Could you check a few things on this model? Use its own coordinates, in mm. A direction names the side the tool comes from. Round coordinates to 2 decimals unless told otherwise and drop trailing zeros. Write each loop counter-clockwise with the first axis right and the second up, starting at its lowest first coordinate (ties: lowest second). Pieces come first, ordered by that corner, then holes. Notation, with made-up numbers: (85, 10.5) -> (107, 10.5) arc R22 ccw to (107, 45.5) -> close; hole circle Ø11 at (74, 52.5). An arc over 180 degrees is marked (long way). Answer in a Markdown table with one row per item.
from build123d import *

# Parameters (mm, degrees)
F0_R     = 4.5
F1_DEPTH = 50
F2_R     = 7.375
F3_DEPTH = 10.1
F4_R     = 37.5
F5_DEPTH = 10


with BuildPart() as f1:
    # F0 (on Top) → F1 (new body)
    with BuildSketch(Plane.XY):
        Circle(F0_R)
    extrude(amount=F1_DEPTH)

    # F2 (on Top) → F3 (join)
    with BuildSketch(Plane.XY):
        Circle(F2_R)
    extrude(amount=-F3_DEPTH)

    # F4 (on face) → F5 (join)
    with BuildSketch(Plane(origin=(0, 0, -10.1), x_dir=(1, 0, 0), z_dir=(0, 0, -1))):
        Circle(F4_R)
    extrude(amount=F5_DEPTH)


solid = f1.part
1) Imagine slicing it at D-D, the plane z = -4. Please give me the cut outline in (x, y) (3 decimals), plus the area to 3 significant figures.
Findings:
| item | result |
|---|---|
| outline | circle Ø14.75 at (0, 0) |
| area | 171 mm^2 |
2) Imagine slicing it at A-A, the plane x = 0. Please give me the cut outline in (y, z) (3 decimals), plus the area to 3 significant figures.
Findings:
| item | result |
|---|---|
| outline | (-37.5, -20.1) -> (37.5, -20.1) -> (37.5, -10.1) -> (7.375, -10.1) -> (7.375, 0) -> (4.5, 0) -> (4.5, 50) -> (-4.5, 50) -> (-4.5, 0) -> (-7.375, 0) -> (-7.375, -10.1) -> (-37.5, -10.1) -> close |
| area | 1,350 mm^2 |
3) Thinking about a two-plate mould opening in X: for faces 3 (the face through (7.034, 2.215, -4.979)), 4 (the face through (-3.4, -3.2, 0)), which applies, +X half, -X half, draft (parallel to the pull), parting line (faces both ways), or undercut?
Findings:
| item | result |
|---|---|
| face 3 | parting line |
| face 4 | draft |
4) For pin 1 (6 mm diameter, centred on x = -10.5, y = 6, fed in from +Z); pin 2 (10 mm diameter, centred on x = 1.5, z = 21, fed in from +Y); pin 3 (2 mm diameter, centred on x = -28.5, z = -12, fed in from -Y), each with a flat end and sliding along its axis, tell me the tip position at first contact or that it passes through.
Findings:
| item | result |
|---|---|
| pin 1 | stops at z = -10.1 |
| pin 2 | stops at y = 4.5 |
| pin 3 | stops at y = -25.5 |
5) For faces 1 (the face through (-1, -1, -20.1)), 2 (the face through (-0.59, 4.46, 24.65)), which set-ups out of +Z, -Z, +X, -X, +Y, -Y let a thin tool reach every point of the face, with its end or its side?
Findings:
| item | result |
|---|---|
| face 1 | -Z, +X, -X, +Y, -Y |
| face 2 | +Z |
6) Imagine slicing it at C-C, the plane z = 43. Please give me the cut outline in (x, y), plus the area to 3 significant figures.
Findings:
| item | result |
|---|---|
| outline | circle Ø9 at (0, 0) |
| area | 63.6 mm^2 |
7) Please list where these lines run through material, in increasing order: line 1 (Z direction, x = -9.5, y = 20.5); line 2 (X direction, y = 6, z = -15); line 3 (X direction, y = 0.5, z = 11).
Findings:
| item | result |
|---|---|
| line 1 | z = -20.1 to -10.1 |
| line 2 | x = -37.02 to 37.02 |
| line 3 | x = -4.47 to 4.47 |
